```python
from build123d import *

# Parameters (mm, degrees)
EXTRUDE_1_DEPTH = 5


with BuildPart() as part:
    # 스케치1 → 보스-돌출1 (new, symmetric)
    with BuildSketch(Plane.XY):
        with BuildLine():
            Line((0, 0), (12.356704667, 0))
            Line((12.356704667, 0), (12.356704667, 3.595174958))
            Line((12.356704667, 3.595174958), (-4.233976366, 3.595174958))
            Line((-4.233976366, 3.595174958), (-3.698633078, -2.084492479))
            ThreePointArc((-3.698633078, -2.084492479), (-12.954718886, -21.310351029), (-31.892829031, -31.141767286))
            ThreePointArc((-31.892829031, -31.141767286), (-55.224518939, -23.45562289), (-62.523719203, 0))
            Line((-62.523719203, 0), (-62.523719203, 3.595174958))
            Line((-62.523719203, 3.595174958), (-73.944795268, 3.595174958))
            Line((-73.944795268, 3.595174958), (-73.944795268, 0))
            Line((-73.944795268, 0), (-66.753336801, 0))
            ThreePointArc((-66.753336801, 0), (-61.985172369, -19.214758492), (-47.563771697, -32.778148135))
            ThreePointArc((-47.563771697, -32.778148135), (-15.773872786, -28.009355466), (0, 0))
        make_face()
    extrude(amount=EXTRUDE_1_DEPTH, both=True)


solid = part.part
```
Geometry check sheet. Reference: the model listing, model coordinates, mm. A direction names the side the tool comes from. Give positions to 0.01 mm unless a question says otherwise; leave off trailing zeros. Loops run counter-clockwise (first coordinate to the right, second up) from the corner with the lowest first, then second, coordinate; pieces in that order, holes last. Notation, with made-up numbers: M 74,54 L 119,54 A35 cw 119,90 Z; hole C -36,40.25 d4. An arc over 180 degrees is marked long. Answer as CSV lines item,"result".
Item 1: Depth check by flat-ended pin: P1, Ø6, axis at x = -48.5, z = 0, coming from the -Y side; P2, Ø5, axis at x = -47, z = 1.5, coming from the -Y side; P3, Ø3.5, axis at x = -71.5, z = 2, coming from the -Y side. Enter the tip coordinate at first touch or a pass-through.
Values:
P1,"stops at y = -33.36"
P2,"stops at y = -33.6"
P3,"stops at y = 0"
Item 2: Release check for a two-part mould opening along Y. For faces 6 (the flat face through (-68, 3.595, 0)), 7 (the flat face through (-28, -31, 5)), 8 (the cylindrical face through (-54.97, -23.71, 0.07)) record: pulls with the +Y half, pulls with the -Y half, needs draft (parallel to the pull), parting line crosses it, or undercut.
Values:
face 6,"pulls with the +Y half"
face 7,"needs draft"
face 8,"undercut"
Item 3: Cross-section at C-C on y = -28.5. Record the cut outline in (x, z), and give its area (3 significant figures).
Values:
outline,"M -54.09,-5 L -48.37,-5 L -48.37,5 L -54.09,5 Z; M -23.14,-5 L -16.5,-5 L -16.5,5 L -23.14,5 Z"
area,"124 mm²"
Item 4: Cross-section at D-D on x = 5. Record the cut outline in (y, z).
Values:
outline,"M 0,-5 L 3.6,-5 L 3.6,5 L 0,5 Z"
Item 5: Access from +Z, -Z, +X, -X, +Y, -Y to the whole of each face (thin tool, end or side, straight path). Record for faces 1 (the cylindrical face through (-16.2, -28.3, 0.1)), 2 (the flat face through (-62.524, 2, 0)), 3 (the flat face through (6, 0, 0)), 4 (the flat face through (-3.97, 0.8, 0.07)), 5 (the flat face through (4, 3.595, 0)).
Values:
face 1,"+Z, -Z, -Y"
face 2,"+Z, -Z, +Y"
face 3,"+Z, -Z, +X, -Y"
face 4,"+Z, -Z"
face 5,"+Z, -Z, +X, -X, +Y"
Item 6: Material ranges on line 1 (X direction, y = -4.5, z = -1); line 2 (X direction, y = -6, z = 4.75); line 3 (Y direction, x = 8, z = 2), recorded low to high.
Values:
line 1,"x = -66.66 to -62.93, -4.1 to -0.54"
line 2,"x = -66.5 to -62.89, -4.44 to -0.85"
line 3,"y = 0 to 3.6"
Item 7: Cross-section at B-B on z = 4. Record the cut outline in (x, y).
Values:
outline,"M -73.94,0 L -66.75,0 A35.04 ccw -47.56,-32.78 A36.61 ccw 0,0 L 12.36,0 L 12.36,3.6 L -4.23,3.6 L -3.7,-2.08 A33.75 cw -31.89,-31.14 A26.83 cw -62.52,0 L -62.52,3.6 L -73.94,3.6 Z"
Item 8: Cross-section at A-A on y = -12. Record the cut outline in (x, z), and give its area (3 significant figures).
Values:
outline,"M -65.18,-5 L -61.9,-5 L -61.9,5 L -65.18,5 Z; M -6.56,-5 L -2.78,-5 L -2.78,5 L -6.56,5 Z"
area,"70.6 mm²"
